from build123d import *

# Parameters (mm, degrees)
SKETCH1_W           = 32
SKETCH1_H           = 31
BOSS_EXTRUDE1_DEPTH = 4
BOSS_EXTRUDE2_DEPTH = 6
SKETCH3_W           = 3
SKETCH3_H           = 4
CUT_EXTRUDE1_DEPTH  = 6
CUT_EXTRUDE6_DEPTH  = 4


with BuildPart() as part:
    # Sketch1 → Boss-Extrude1 (new body)
    with BuildSketch(Plane(origin=(0, 0, 0), x_dir=(1, 0, 0), z_dir=(0, 1, 0))):
        Rectangle(SKETCH1_W, SKETCH1_H)
    extrude(amount=BOSS_EXTRUDE1_DEPTH)

    # Sketch2 → Boss-Extrude2 (add)
    with BuildSketch(Plane(origin=(0, 4, 0), x_dir=(1, 0, 0), z_dir=(0, 1, 0))):
        Polygon((-16, 15.5), (-16, -15.5), (0, -15.5), (0, -11.5), (-12, -11.5), (-12, 11.5), (0, 11.5), (0, 15.5), align=None)
    extrude(amount=BOSS_EXTRUDE2_DEPTH)

    # Sketch3 → Cut-Extrude1 (cut)
    with BuildSketch(Plane(origin=(0, 10, 0), x_dir=(1, 0, 0), z_dir=(0, 1, 0))):
        with Locations((-5.5, 13.5)):
            Rectangle(SKETCH3_W, SKETCH3_H)
    extrude(amount=-CUT_EXTRUDE1_DEPTH, mode=Mode.SUBTRACT)

    # Sketch4 → Cut-Extrude6 (cut)
    with BuildSketch(Plane(origin=(0, 4, 0), x_dir=(0.7071067811864886, 0, -0.7071067811866065), z_dir=(0, 1, 0))):
        with BuildLine():
            Line((14, 2), (2.449489743, 2.5))
            ThreePointArc((2.449489743, 2.5), (3.226702194, 1.355873501), (3.5, 0))
            ThreePointArc((3.5, 0), (3.226702194, -1.355873501), (2.449489743, -2.5))
            Line((2.449489743, -2.5), (14, -2))
            ThreePointArc((14, -2), (15.414213562, -1.414213562), (16, 0))
            ThreePointArc((16, 0), (15.414213562, 1.414213562), (14, 2))
        make_face()
        with BuildLine():
            ThreePointArc((3.5, 0), (3.226702194, 1.355873501), (2.449489743, 2.5))
            ThreePointArc((2.449489743, 2.5), (-3.5, 0), (2.449489743, -2.5))
            ThreePointArc((2.449489743, -2.5), (3.226702194, -1.355873501), (3.5, 0))
        make_face()
    extrude(amount=-CUT_EXTRUDE6_DEPTH, mode=Mode.SUBTRACT)


solid = part.part
Input: part model. Units: mm. Frame: model coordinates. A direction names the side the tool comes from. Round coordinates to 2 decimals unless told otherwise and drop trailing zeros. Write each loop counter-clockwise with the first axis right and the second up, starting at its lowest first coordinate (ties: lowest second). Pieces come first, ordered by that corner, then holes.
1) Contact query for flat-ended pins moving along their axis: P1, Ø2, axis at y = 7, z = 14, coming from the +X side; P2, Ø8, axis at x = 0, z = 0, coming from the +Y side. Output: stop coordinate, or through.
2) Cut plane D-D (x = 4). Return the cut outline in (y, z).
3) Cut plane B-B (z = -0.5). Return the cut outline in (x, y), then the cut area to 3 significant figures.
4) Draft query along Z for faces 4 (the flat face through (-16, 5, 0)), 5 (the flat face through (-10, 7, -11.5)), 6 (the flat face through (-4, 4, 15.5)). Return one class per face: pulls with the +Z half, pulls with the -Z half, needs draft (parallel to the pull), parting line crosses it, or undercut.
5) Reachability of faces 1 (the flat face through (-6, 7, 11.5)), 2 (the flat face through (7.352, 2.028, -4.165)), 3 (the flat face through (0, 7, -13)) from +Z, -Z, +X, -X, +Y, -Y: full face, straight path, thin tool, end or side. Return the list, or none.
6) Ray query, L1, parallel to Y at x = -6, z = 1; L2, parallel to Z at x = -0.5, y = 6; L3, parallel to X at y = 7.5, z = 13. Return the intervals inside material, ascending.
7) Cut plane C-C (y = 2.5). Return the cut outline in (x, z).
8) Cut plane A-A (y = 7.75). Return the cut outline in (x, z), then the cut area to 3 significant figures.
Geometry says:
1. P1: stops at x = 0
1. P2: stops at y = 4
2. outline: (0, -15.5) - (4, -15.5) - (4, -7.2) - (0, -7.2) - close; (0, -0.51) - (4, -0.51) - (4, 15.5) - (0, 15.5) - close
3. outline: (-16, 0) - (-3.46, 0) - (-3.46, 4) - (-12, 4) - (-12, 10) - (-16, 10) - close; (3.99, 0) - (16, 0) - (16, 4) - (3.99, 4) - close
3. area: 122 mm2
4. face 4: needs draft
4. face 5: undercut
4. face 6: pulls with the +Z half
5. face 1: +X, +Y
5. face 2: +Y, -Y
5. face 3: +Z, -Z, +X, +Y
6. L1: y = 0 to 4
6. L2: z = -15.5 to -11.5, 11.5 to 15.5
6. L3: x = -16 to 0
7. outline: (-16, -15.5) - (16, -15.5) - (16, 15.5) - (-16, 15.5) - close; hole (-0.04, -3.5) - (8.49, -11.31) arc R2 ccw to (11.31, -8.49) - (3.5, 0.04) arc R3.5 ccw (long way) to start
8. outline: (-16, -15.5) - (-7, -15.5) - (-7, -11.5) - (-12, -11.5) - (-12, 11.5) - (0, 11.5) - (0, 15.5) - (-16, 15.5) - close; (-4, -15.5) - (0, -15.5) - (0, -11.5) - (-4, -11.5) - close
8. area: 208 mm2
